Geometry: final body of the model. Coordinates: model frame, mm. Give positions to 0.01 mm unless a question says otherwise; leave off trailing zeros. Write each loop counter-clockwise with the first axis right and the second up, starting at its lowest first coordinate (ties: lowest second). Pieces come first, ordered by that corner, then holes. Notation, with made-up numbers: (64, 8) -> (87, 8) arc R9 ccw to (87, 21) -> close; hole circle Ø8 at (-17, -38.5). An arc over 180 degrees is marked (long way). Answer in a Markdown table with one row per item. Add a question column.
from build123d import *

# Parameters (mm, degrees)
F0_W     = 304.8
F0_H     = 304.8
F0_R     = 3.175
F0_R_2   = 2.413
F0_W_2   = 185.928
F0_H_2   = 185.928
F1_DEPTH = 2.778125


with BuildPart() as f1:
    # F0 (on Front) → F1 (new body)
    with BuildSketch(Plane.XZ):
        Rectangle(F0_W, F0_H)
        with Locations((-139.7, -139.7)):
            Circle(F0_R, mode=Mode.SUBTRACT)
        with Locations((-50.8, -98.552)):
            Circle(F0_R_2, mode=Mode.SUBTRACT)
        with Locations((50.8, -98.552)):
            Circle(F0_R_2, mode=Mode.SUBTRACT)
        with Locations((139.7, -139.7)):
            Circle(F0_R, mode=Mode.SUBTRACT)
        with Locations((-139.7, 139.7)):
            Circle(F0_R, mode=Mode.SUBTRACT)
        with Locations((-76.2, 98.552)):
            Circle(F0_R_2, mode=Mode.SUBTRACT)
        Rectangle(F0_W_2, F0_H_2, mode=Mode.SUBTRACT)
        with Locations((0, 98.552)):
            Circle(F0_R_2, mode=Mode.SUBTRACT)
        with Locations((76.2, 98.552)):
            Circle(F0_R_2, mode=Mode.SUBTRACT)
        with Locations((139.7, 139.7)):
            Circle(F0_R, mode=Mode.SUBTRACT)
    extrude(amount=F1_DEPTH)


solid = f1.part
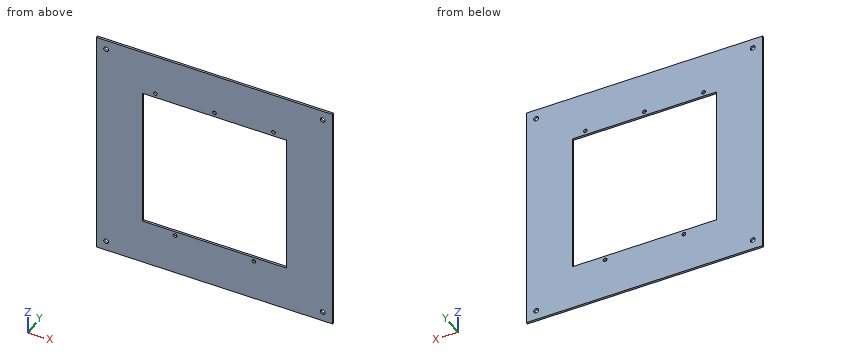
Q1. Line query: probe 1 along X at (y, z) = (-1.9, 139.7) (3 decimals); probe 2 along Z at (x, y) = (-76.2, -2.15) (3 decimals). Output: solid intervals per line, ascending. Write a range as from..to.
Q2. Section C-C on y = -0.45. Count the separate pieces of the cut face and the enclosed holes in it, and give its area (3 significant figures).
Q3. Section B-B on x = -37. Return loops of the section in (y, z), and give its area (3 significant figures).
Q4. Section A-A on z = 37.5. Return loops of the section in (x, y).
Q5. Contact query for flat-ended pins moving along their axis: pin 1 Ø3 at (x, z) = (-76.2, 98.552) entering from +Y; pin 2 Ø7.5 at (x, z) = (50.8, -98.552) entering from -Y. Output: stop coordinate, or through.
Checks:
| question | item | result |
|---|---|---|
| 1 | probe 1 | -152.4..-142.875, -136.525..136.525, 142.875..152.4 |
| 1 | probe 2 | -152.4..-92.964, 92.964..96.139, 100.965..152.4 |
| 2 | separate pieces | 1 |
| 2 | enclosed holes | 10 |
| 2 | area | 58,100 mm^2 |
| 3 | outline | (-2.78, -152.4) -> (0, -152.4) -> (0, -92.96) -> (-2.78, -92.96) -> close; (-2.78, 92.96) -> (0, 92.96) -> (0, 152.4) -> (-2.78, 152.4) -> close |
| 3 | area | 330 mm^2 |
| 4 | outline | (-152.4, -2.78) -> (-92.96, -2.78) -> (-92.96, 0) -> (-152.4, 0) -> close; (92.96, -2.78) -> (152.4, -2.78) -> (152.4, 0) -> (92.96, 0) -> close |
| 5 | pin 1 | through |
| 5 | pin 2 | y = -2.78 |
